Source: CAD feature listing. Evaluate the final solid. Frame: model axes, mm. Give positions to 0.01 mm unless a question says otherwise; leave off trailing zeros. Order: outer loops, then holes, each group sorted by start corner. A loop starts at its lowest first (then second) coordinate and runs counter-clockwise, first axis right, second up. Notation, with made-up numbers: (60.5, 0) - (81.5, 0) arc R26 cw to (81.5, 38) - close; hole circle Ø4 at (-16.5, 62.25). An arc over 180 degrees is marked (long way). Write each question's results on one line, items separated by ' | '. Start each with the question number.
Item 1: Section B-B on z = 0. Output: boundary loops of the cut face in (x, y), and give its area (3 significant figures).
Item 2: Section C-C on y = 3.15. Output: boundary loops of the cut face in (x, z), and give its area (3 significant figures).
Item 3: Contact query for a flat-ended pin moving along its axis: pin 1 Ø2 at (y, z) = (1, 7) entering from +X. Output: stop coordinate, or through.
Item 4: Section D-D on y = 4.2. Output: boundary loops of the cut face in (x, z), and give its area (3 significant figures).
Item 5: Line query: line 1 along X through (y, z) = (2.75, 0); line 2 along X through (y, z) = (1.6, -3.5); line 3 along Z through (x, y) = (-3, 1.4). Output: solid intervals per line, ascending.
Item 6: Mould query, pull axis X, two halves, no side actions, for faces 1 (the cylindrical face through (3.905, 2.465, -0.867)), 2 (the flat face through (3, 0, -3)), 3 (the cylindrical face through (7.81, 2.22, -1.73)). Classes: released by +X, released by -X, zero draft, split by the parting line, or undercut.
Item 7: Section A-A on x = 0. Output: boundary loops of the cut face in (y, z).
```python
from build123d import *

# Parameters (mm, degrees)
CHAMFER_1_SIZE = 0.5
CHAMFER_2_SIZE = 0.2


with BuildPart() as part:
    # 草图1 → 旋转1 (revolve)
    with BuildSketch(Plane.XY, mode=Mode.PRIVATE) as revolve_1_sk:
        Polygon((-4, 0), (-8, 0), (-8, 3.9), (-9, 3.9), (-9, 5), (-4, 5), align=None)
    revolve(revolve_1_sk.sketch.rotate(Axis((0, 10.75638676, 0), (0, -1, 0)), 270), axis=Axis((0, 10.75638676, 0), (0, -1, 0)))

    # 倒角1
    chamfer_1_edges = [part.edges().sort_by_distance(p)[0] for p in [
        (0, 0, -8),
    ]]
    chamfer(chamfer_1_edges, length=CHAMFER_1_SIZE)

    # 倒角2
    chamfer_2_edges = [part.edges().sort_by_distance(p)[0] for p in [
        (0, 5, -9),
    ]]
    chamfer(chamfer_2_edges, length=CHAMFER_2_SIZE)


solid = part.part
```
Evaluation:
1) outline: (-9, 3.9) - (-8, 3.9) - (-8, 0.5) - (-7.5, 0) - (-4, 0) - (-4, 5) - (-8.8, 5) - (-9, 4.8) - close; (4, 0) - (7.5, 0) - (8, 0.5) - (8, 3.9) - (9, 3.9) - (9, 4.8) - (8.8, 5) - (4, 5) - close | area: 41.9 mm^2
2) outline: circle Ø16 at (0, 0); hole circle Ø8 at (0, 0) | area: 151 mm^2
3) pin 1: stops at x = 5.29
4) outline: circle Ø18 at (0, 0); hole circle Ø8 at (0, 0) | area: 204 mm^2
5) line 1: x = -8 to -4, 4 to 8 | line 2: x = -7.19 to -1.94, 1.94 to 7.19 | line 3: z = -7.42 to -2.65, 2.65 to 7.42
6) face 1: undercut | face 2: zero draft | face 3: split by the parting line
7) outline: (0, -7.5) - (0.5, -8) - (3.9, -8) - (3.9, -9) - (4.8, -9) - (5, -8.8) - (5, -4) - (0, -4) - close; (0, 4) - (5, 4) - (5, 8.8) - (4.8, 9) - (3.9, 9) - (3.9, 8) - (0.5, 8) - (0, 7.5) - close
